Design review of the part shown in the three views and the two pictorial views. Dimensions are in mm from the part's minimum x, y and z. Coordinates: 2 decimals unless noted, no trailing zeros. Loops run counter-clockwise (first coordinate to the right, second up) from the corner with the lowest first, then second, coordinate; pieces in that order, holes last. Notation, with made-up numbers: (-20.75, 19.5) -> (21.25, 19.5) arc R4 cw to (21.25, 26.5) -> close; hole circle Ø7 at (10.5, 23.5). An arc over 180 degrees is marked (long way). One line per item, written item: value. Start each with the question number.
1. For probe 1 along Y at (x, z) = (27, 4.7); probe 2 along Y at (x, z) = (27, 3.15); probe 3 along Y at (x, z) = (42.5, 3.75) (1 decimal), list the stretches that pass through material, from the lowest coordinate up.
2. Add section A-A on y = 27. Write out the cut boundary in (x, z), plus the area to 3 significant figures.
3. Add section B-B on z = 3.25. Give the number of separate pieces and of enclosed holes in the cut face, plus the area to 3 significant figures.
4. Draft analysis for pull direction Y (two halves, no side actions). For the marked faces 1, 2 and 3, state which applies: pulls with the +Y half, pulls with the -Y half, needs draft (parallel to the pull), parting line crosses it, or undercut.
5. Insertion check: pin 1 (3 mm diameter, centred on x = 44.5, y = 17, fed in from +Z); pin 2 (3 mm diameter, centred on y = 42, z = 0.5, fed in from +X); pin 3 (1 mm diameter, centred on x = 46.5, y = 12, fed in from -Z); pin 4 (1.5 mm diameter, centred on y = 8.5, z = 5, fed in from -X) (1 decimal). Each pin has a flat end and moves straight along its axis. Give the tip position at first contact, or say it passes through.
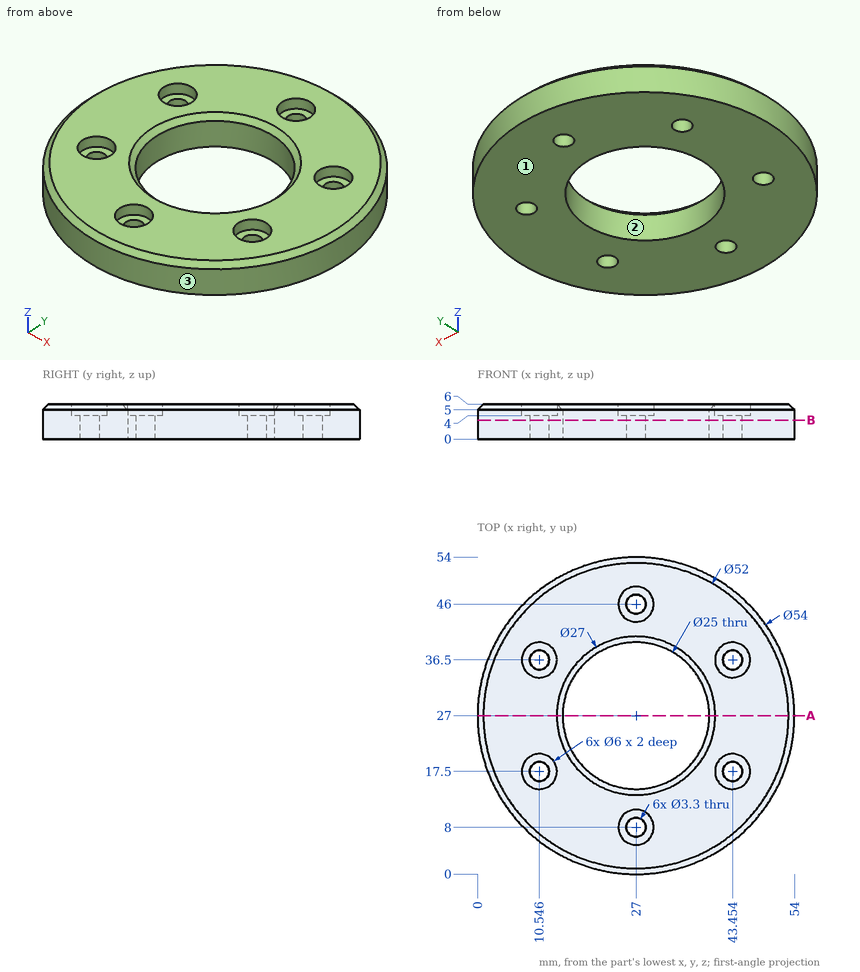
Worked answers:
1. probe 1: y = 0 to 5, 11 to 14.5, 39.5 to 43, 49 to 54
1. probe 2: y = 0 to 6.35, 9.65 to 14.5, 39.5 to 44.35, 47.65 to 54
1. probe 3: y = 4.9 to 16.2, 18.8 to 35.2, 37.8 to 49.1
2. outline: (0, 0) -> (14.5, 0) -> (14.5, 5) -> (13.5, 6) -> (1, 6) -> (0, 5) -> close; (39.5, 0) -> (54, 0) -> (54, 5) -> (53, 6) -> (40.5, 6) -> (39.5, 5) -> close
2. area: 172 mm²
3. separate pieces: 1
3. enclosed holes: 7
3. area: 1,750 mm²
4. face 1: needs draft
4. face 2: undercut
4. face 3: parting line crosses it
5. pin 1: stops at z = 4
5. pin 2: stops at x = 50.38
5. pin 3: stops at z = 0
5. pin 4: stops at x = 6.7
